Design review of the part shown in the three views and the two pictorial views. Dimensions are in mm from the part's minimum x, y and z. Coordinates: 2 decimals unless noted, no trailing zeros. Order: outer loops, then holes, each group sorted by start corner. A loop starts at its lowest first (then second) coordinate and runs counter-clockwise, first axis right, second up. Notation, with made-up numbers: (43.25, 31) - (53.25, 31) arc R19 cw to (53.25, 40) - close; hole circle Ø10 at (38, 69). An arc over 180 degrees is marked (long way). One line per item, written item: value. Start each with the question number.
(1) Consider section A-A on x = 3.5. Write out the cut boundary in (y, z), then the cut area to 3 significant figures.
(2) Consider section B-B on z = 3.5. Write out the cut boundary in (x, y), then the cut area to 3 significant figures.
(3) To check wall thickness, follow line 1 along Y through (x, z) = (3, 1.9); line 2 along X through (y, z) = (141, 1.15); line 3 along Y through (x, z) = (17.75, 3.5). State the ranges of each line that lie inside material, in increasing order.
(4) Clearance check with flat-ended pins moving along their axes: pin 1 (3 mm diameter, centred on x = 15, z = 1.5, fed in from -Y); pin 2 (1.6 mm diameter, centred on y = 74, z = 3, fed in from -X); pin 3 (3 mm diameter, centred on x = 2, z = 2, fed in from -Y). State where each tip first meets the part, or that it passes through.
(5) Consider section C-C on y = 74. Write out the cut boundary in (x, z), then the cut area to 3 significant figures.
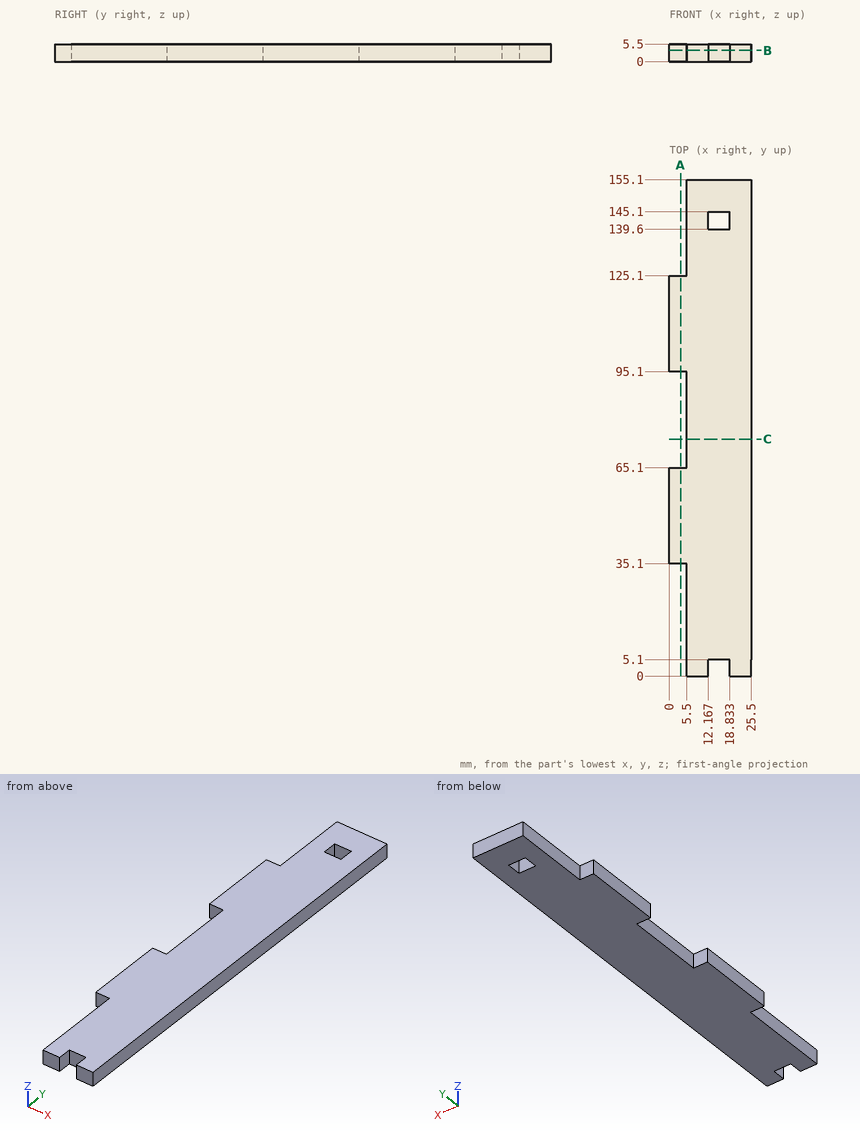
Geometry check:
1. outline: (35.1, 0) - (65.1, 0) - (65.1, 5.5) - (35.1, 5.5) - close; (95.1, 0) - (125.1, 0) - (125.1, 5.5) - (95.1, 5.5) - close
1. area: 330 mm^2
2. outline: (0, 35.1) - (5.5, 35.1) - (5.5, 0) - (12.17, 0) - (12.17, 5.1) - (18.83, 5.1) - (18.83, 0) - (25.5, 0) - (25.5, 155.1) - (5.5, 155.1) - (5.5, 125.1) - (0, 125.1) - (0, 95.1) - (5.5, 95.1) - (5.5, 65.1) - (0, 65.1) - close; hole (12.17, 139.6) - (18.83, 139.6) - (18.83, 145.1) - (12.17, 145.1) - close
2. area: 3,360 mm^2
3. line 1: y = 35.1 to 65.1, 95.1 to 125.1
3. line 2: x = 5.5 to 12.17, 18.83 to 25.5
3. line 3: y = 5.1 to 139.6, 145.1 to 155.1
4. pin 1: stops at y = 5.1
4. pin 2: stops at x = 5.5
4. pin 3: stops at y = 35.1
5. outline: (5.5, 0) - (25.5, 0) - (25.5, 5.5) - (5.5, 5.5) - close
5. area: 110 mm^2
